Study the drawing (mm; zero at the part's minimum x, y, z) and answer. Give positions to 0.01 mm unless a question says otherwise; leave off trailing zeros. Order: outer loops, then holes, each group sorted by start corner. A loop starts at its lowest first (then second) coordinate and runs counter-clockwise, first axis right, second up.
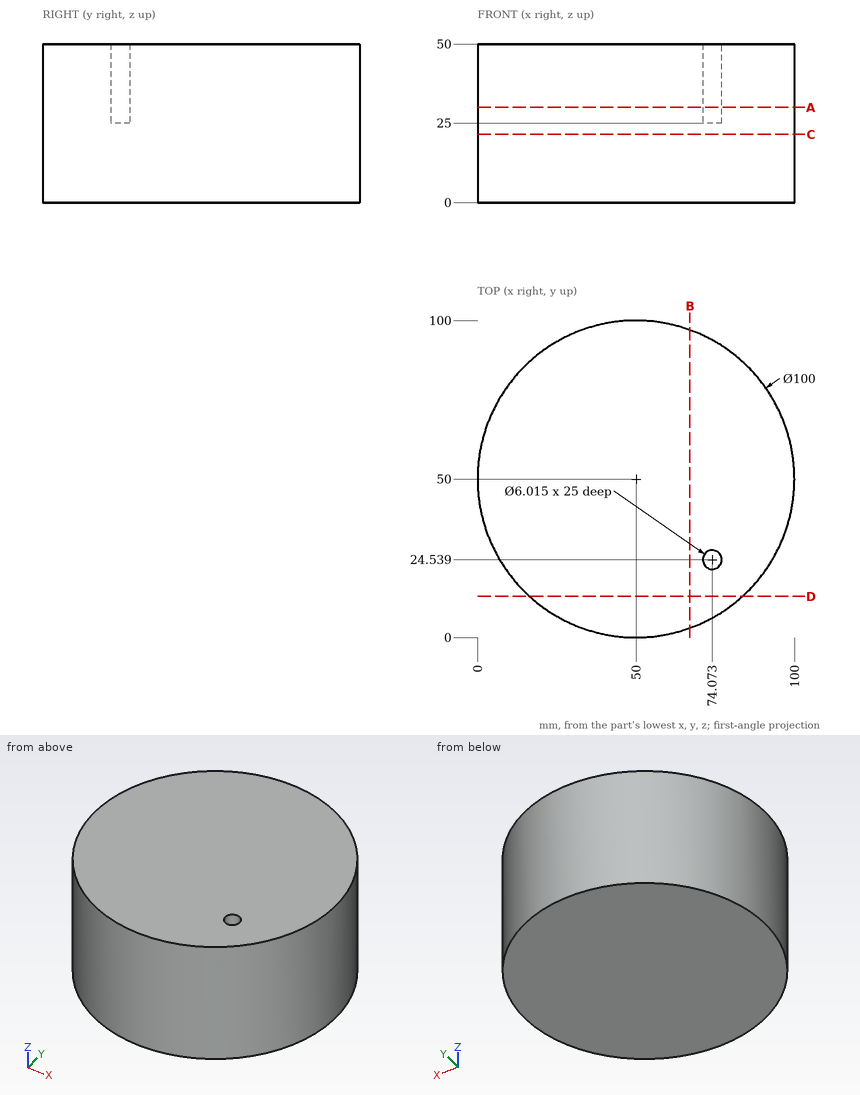
1) Given P1, Ø3, axis at y = 35, z = 29.5, coming from the +X side; P2, Ø2, axis at y = 16.5, z = 41.5, coming from the -X side; P3, Ø9.5, axis at x = 74.07, y = 24.54, coming from the +Z side; P4, Ø10, axis at x = 64.5, z = 17.5, coming from the -Y side, each flat-ended and moving along its own axis, determine where each tip first touches the part or whether it passes through.
Geometry says:
P1: stops at x = 98.14
P2: stops at x = 12
P3: stops at z = 50
P4: stops at y = 0.91
2) Find section B-B (x = 67). Write down the section's boundary in (y, z).
Geometry says:
outline: (2.98, 0) - (97.02, 0) - (97.02, 50) - (2.98, 50) - close
3) Straight lines are drawn through the part: probe 1 along Y at (x, z) = (51, 40.5); probe 2 along X at (y, z) = (75.5, 21.5); probe 3 along Y at (x, z) = (9.5, 3) (1 decimal). For each, find the intervals that lie inside material, in ascending order.
Geometry says:
probe 1: y = 0.01 to 99.99
probe 2: x = 6.99 to 93.01
probe 3: y = 20.7 to 79.3
4) Find section C-C (z = 21.5). Write down the section's boundary in (x, y), then the cut area to 3 significant figures.
Geometry says:
outline: circle Ø100 at (50, 50)
area: 7,850 mm2
5) Find section D-D (y = 13). Write down the section's boundary in (x, z).
Geometry says:
outline: (16.37, 0) - (83.63, 0) - (83.63, 50) - (16.37, 50) - close
6) Find section A-A (z = 30). Write down the section's boundary in (x, y) (1 decimal), then the cut area to 3 significant figures.
Geometry says:
outline: circle Ø100 at (50, 50); hole circle Ø6 at (74.1, 24.5)
area: 7,830 mm2
